Input: part model. Units: mm. Frame: model coordinates. Face numbers are marked on the shaded views. A direction names the side the tool comes from. Round coordinates to 2 decimals unless told otherwise and drop trailing zeros. Loops run counter-clockwise (first coordinate to the right, second up) from the corner with the lowest first, then second, coordinate; pieces in that order, holes last.
(1) Draft query along Y for the marked faces 5, 6 and 7. Return one class per face: released by +Y, released by -Y, zero draft, split by the parting line, or undercut.
(2) Cut plane A-A, the plane z = 14.5. Output: boundary loops of the cut face in (x, y) (3 decimals).
(3) Line query: line 1 (Z direction, x = 4, y = -2.5); line 2 (X direction, y = 0.5, z = 17); line 3 (X direction, y = -6.25, z = 2.5). Output: solid intervals per line, ascending.
(4) Access query for the marked faces 1, 2, 3 and 4. Directions: +Z, -Z, +X, -X, +Y, -Y. A direction counts if a zero-diameter tool reaches every point of the face in a straight line with its end or side. Return the directions, or none.
(5) Cut plane D-D, the plane z = 2. Output: boundary loops of the cut face in (x, y), and give its area (3 significant figures).
(6) Cut plane B-B, the plane x = 4.5. Output: boundary loops of the cut face in (y, z), and give its area (3 significant figures).
(7) First-contact query: pin 1 Ø2 at (y, z) = (5, 16) entering from -X; pin 2 Ø2 at (y, z) = (3, 6.5) entering from +X; pin 3 Ø1.1 at (y, z) = (0.5, 15) entering from -X; pin 4 Ø4 at (y, z) = (1, 18.5) entering from +X. Flat tips, straight axial feed; report the tip coordinate or a pass-through.
(8) Cut plane C-C, the plane x = 2.5. Output: boundary loops of the cut face in (y, z).
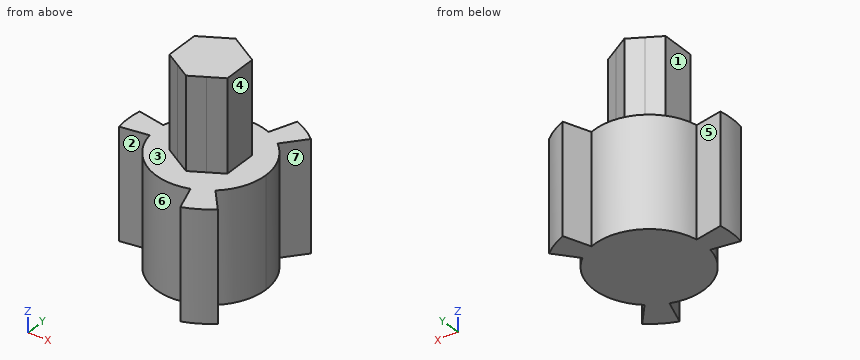
from build123d import *

# Parameters (mm, degrees)
F1_DEPTH = 12
F3_DEPTH = 10


with BuildPart() as f1:
    # F0 (on Top) → F1 (new body)
    with BuildSketch(Plane.XY):
        with BuildLine():
            Line((-5.9160797831, 1), (-8.8741196746, 1.5))
            ThreePointArc((-8.8741196746, 1.5), (-9, 0), (-8.8741196746, -1.5))
            Line((-8.8741196746, -1.5), (-5.9160797831, -1))
            ThreePointArc((-5.9160797831, -1), (-6, 0), (-5.9160797831, 1))
        make_face()
        with BuildLine():
            ThreePointArc((6, 0), (5.4280787943, 2.5565524839), (3.8213464657, 4.6257227748))
            ThreePointArc((3.8213464657, 4.6257227748), (3, 5.1961524227), (2.0953202009, 5.6222445034))
            ThreePointArc((2.0953202009, 5.6222445034), (-2.9984724458, 5.1970340572), (-5.9160797831, 1))
            ThreePointArc((-5.9160797831, 1), (-6, 0), (-5.9160797831, -1))
            ThreePointArc((-5.9160797831, -1), (-3.0422841899, -5.1715091519), (2, -5.6568542495))
            ThreePointArc((2, -5.6568542495), (3, -5.1961524227), (3.8989794856, -4.5604779323))
            ThreePointArc((3.8989794856, -4.5604779323), (5.4494897428, -2.5105898796), (6, 0))
        make_face()
        with BuildLine():
            Line((3.8213464657, 4.6257227748), (5.7320196986, 6.9385841621))
            ThreePointArc((5.7320196986, 6.9385841621), (4.5, 7.7942286341), (3.1429803014, 8.433366755))
            Line((3.1429803014, 8.433366755), (2.0953202009, 5.6222445034))
            ThreePointArc((2.0953202009, 5.6222445034), (3, 5.1961524227), (3.8213464657, 4.6257227748))
        make_face()
        with BuildLine():
            ThreePointArc((3, -8.4852813742), (4.5, -7.7942286341), (5.8484692283, -6.8407168985))
            Line((5.8484692283, -6.8407168985), (3.8989794856, -4.5604779323))
            ThreePointArc((3.8989794856, -4.5604779323), (3, -5.1961524227), (2, -5.6568542495))
            Line((2, -5.6568542495), (3, -8.4852813742))
        make_face()
    extrude(amount=F1_DEPTH)

    # F2 (on face) → F3 (join)
    with BuildSketch(Plane.XY.offset(12)):
        with BuildLine():
            ThreePointArc((1.5750000902, -2.7279799699), (2.727980048, -1.5749999549), (3.15, 0))
            ThreePointArc((3.15, 0), (2.7279800298, 1.5749999864), (1.5750000272, 2.7279800062))
            ThreePointArc((1.5750000272, 2.7279800062), (1.5e-08, 3.15), (-1.5750000013, 2.7279800212))
            ThreePointArc((-1.5750000013, 2.7279800212), (-2.7279800223, 1.5749999993), (-3.15, 0))
            ThreePointArc((-3.15, 0), (-2.7279800223, -1.5749999993), (-1.5750000013, -2.7279800212))
            ThreePointArc((-1.5750000013, -2.7279800212), (5.13e-08, -3.15), (1.5750000902, -2.7279799699))
        make_face()
        with BuildLine():
            Line((3.15, -1.8186533479), (3.15, 0))
            ThreePointArc((3.15, 0), (2.727980048, -1.5749999549), (1.5750000902, -2.7279799699))
            Line((1.5750000902, -2.7279799699), (3.15, -1.8186533479))
        make_face()
        with BuildLine():
            ThreePointArc((1.5750000272, 2.7279800062), (2.7279800298, 1.5749999864), (3.15, 0))
            Line((3.15, 0), (3.15, 1.8186533479))
            Line((3.15, 1.8186533479), (1.5750000272, 2.7279800062))
        make_face()
        with BuildLine():
            ThreePointArc((-1.5750000013, 2.7279800212), (1.5e-08, 3.15), (1.5750000272, 2.7279800062))
            Line((1.5750000272, 2.7279800062), (0, 3.6373066959))
            Line((0, 3.6373066959), (-1.5750000013, 2.7279800212))
        make_face()
        with BuildLine():
            Line((0, -3.6373066959), (1.5750000902, -2.7279799699))
            ThreePointArc((1.5750000902, -2.7279799699), (5.13e-08, -3.15), (-1.5750000013, -2.7279800212))
            Line((-1.5750000013, -2.7279800212), (0, -3.6373066959))
        make_face()
        with BuildLine():
            ThreePointArc((-3.15, 0), (-2.7279800223, 1.5749999993), (-1.5750000013, 2.7279800212))
            Line((-1.5750000013, 2.7279800212), (-3.15, 1.8186533479))
            Line((-3.15, 1.8186533479), (-3.15, 0))
        make_face()
        with BuildLine():
            Line((-3.15, -1.8186533479), (-1.5750000013, -2.7279800212))
            ThreePointArc((-1.5750000013, -2.7279800212), (-2.7279800223, -1.5749999993), (-3.15, 0))
            Line((-3.15, 0), (-3.15, -1.8186533479))
        make_face()
    extrude(amount=F3_DEPTH)


solid = f1.part
Reported:
1. face 5: released by +Y
1. face 6: released by -Y
1. face 7: undercut
2. outline: (-3.15, -1.819) - (0, -3.637) - (3.15, -1.819) - (3.15, 1.819) - (0, 3.637) - (-3.15, 1.819) - close
3. line 1: z = 0 to 12
3. line 2: x = -3.15 to 3.15
3. line 3: x = 2.21 to 5.34
4. face 1: +Z, -X, +Y, -Y
4. face 2: +Z, -Z, -Y
4. face 3: +Z
4. face 4: +Z, +X, +Y, -Y
5. outline: (-8.87, -1.5) - (-5.92, -1) arc R6 ccw to (2, -5.66) - (3, -8.49) arc R9 ccw to (5.85, -6.84) - (3.9, -4.56) arc R6 ccw to (3.82, 4.63) - (5.73, 6.94) arc R9 ccw to (3.14, 8.43) - (2.1, 5.62) arc R6 ccw to (-5.92, 1) - (-8.87, 1.5) arc R9 ccw to start
5. area: 136 mm2
6. outline: (-7.79, 0) - (-5.26, 0) - (-5.26, 12) - (-7.79, 12) - close; (-3.97, 0) - (3.97, 0) - (3.97, 12) - (-3.97, 12) - close; (5.45, 0) - (7.79, 0) - (7.79, 12) - (5.45, 12) - close
6. area: 154 mm2
7. pin 1: passes through
7. pin 2: stops at x = 5.66
7. pin 3: stops at x = -3.15
7. pin 4: stops at x = 3.15
8. outline: (-7.07, 0) - (6.71, 0) - (6.71, 12) - (2.19, 12) - (2.19, 22) - (-2.19, 22) - (-2.19, 12) - (-7.07, 12) - close
